Build history of the part. All positions in model axes, mm. Coordinates: 2 decimals unless noted, no trailing zeros. Write each loop counter-clockwise with the first axis right and the second up, starting at its lowest first coordinate (ties: lowest second). Pieces come first, ordered by that corner, then holes. Notation, with made-up numbers: (30.25, 15.5) -> (74.25, 15.5) arc R22 cw to (74.25, 53.5) -> close; hole circle Ø11 at (-35, 28.25). An arc over 180 degrees is marked (long way). Write each question's results on one line, items separated by ' | '. Start each with the question number.
Q1. Saw through at B-B on x = 30. Give the cut face in (y, z).
Q2. Drop a flat-ended pin along its axis: pin 1 Ø3 at (x, z) = (-30, 0) entering from -Y. Give the stop position or say it passes through.
Q3. Drill centre lines: line 1 (X direction, y = 7.5, z = 0); line 2 (Z direction, x = 30, y = 6.25); line 3 (Z direction, x = -28, y = 6). Where is each one in solid material? Low to high.
Q4. Two-plate mould, pull along Z, no slides. Class faces 1 (the face through (27.62, 5.07, -0.1)), 2 (the face through (-1, 5, 25)), 3 (the face through (-40, 5, 0)): released by +Z, released by -Z, zero draft, split by the parting line, or undercut.
Q5. Saw through at A-A on z = 0. Give the cut face in (x, y), and give its area (3 significant figures).
from build123d import *

# Parameters (mm, degrees)
SKETCH1_W           = 80
SKETCH1_H           = 50
BOSS_EXTRUDE1_DEPTH = 10
SKETCH2_R           = 2.38125
CUT_EXTRUDE1_DEPTH  = 10


with BuildPart() as part:
    # Sketch1 → Boss-Extrude1 (new body)
    with BuildSketch(Plane(origin=(0, 0, 0), x_dir=(1, 0, 0), z_dir=(0, 1, 0))):
        Rectangle(SKETCH1_W, SKETCH1_H)
    extrude(amount=BOSS_EXTRUDE1_DEPTH)

    # Sketch2 → Cut-Extrude1 (cut)
    with BuildSketch(Plane(origin=(0, 10, 0), x_dir=(1, 0, 0), z_dir=(0, 1, 0))):
        with Locations((-30, 0)):
            Circle(SKETCH2_R)
        with Locations((30, 0)):
            Circle(SKETCH2_R)
    extrude(amount=-CUT_EXTRUDE1_DEPTH, mode=Mode.SUBTRACT)


solid = part.part
Returned:
1) outline: (0, -25) -> (10, -25) -> (10, -2.38) -> (0, -2.38) -> close; (0, 2.38) -> (10, 2.38) -> (10, 25) -> (0, 25) -> close
2) pin 1: passes through
3) line 1: x = -40 to -32.38, -27.62 to 27.62, 32.38 to 40 | line 2: z = -25 to -2.38, 2.38 to 25 | line 3: z = -25 to -1.29, 1.29 to 25
4) face 1: undercut | face 2: released by +Z | face 3: zero draft
5) outline: (-40, 0) -> (-32.38, 0) -> (-32.38, 10) -> (-40, 10) -> close; (-27.62, 0) -> (27.62, 0) -> (27.62, 10) -> (-27.62, 10) -> close; (32.38, 0) -> (40, 0) -> (40, 10) -> (32.38, 10) -> close | area: 705 mm2
